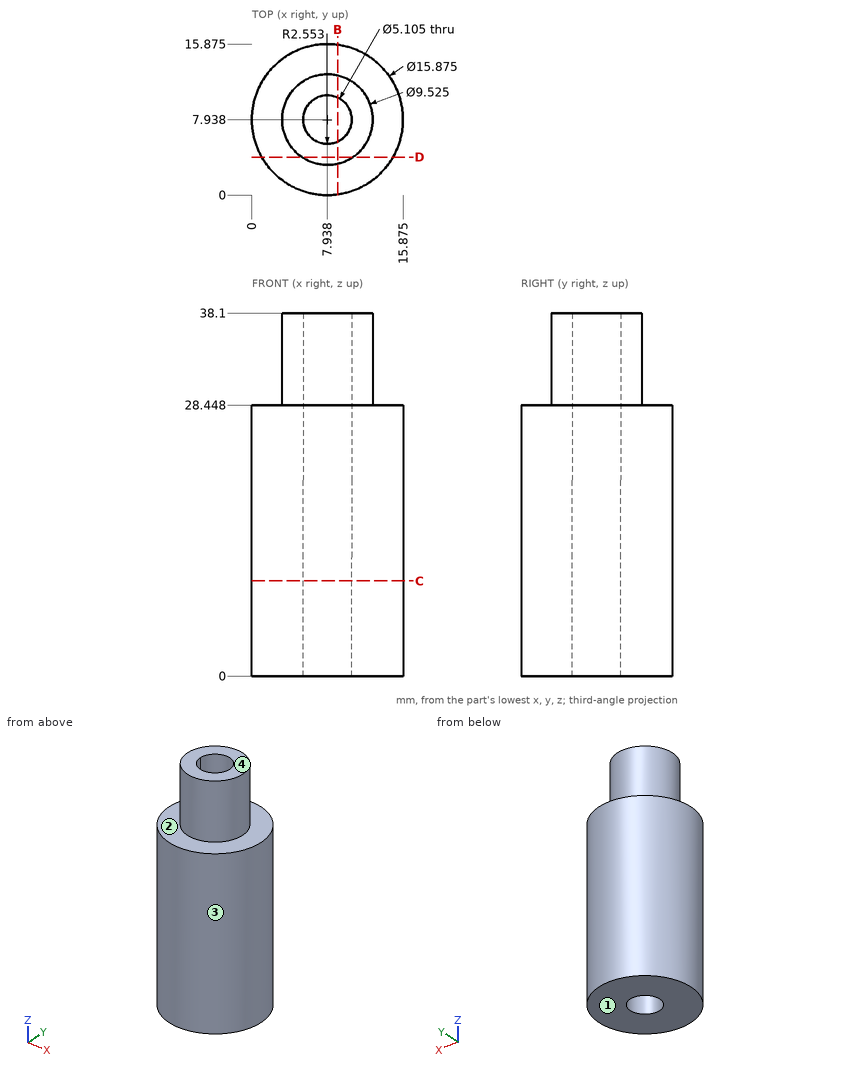
Part print with two shaded views. Sizes in mm from the minimum x, y, z corner. A direction names the side the tool comes from. Coordinates: 2 decimals unless noted, no trailing zeros. Write each loop counter-clockwise with the first axis right and the second up, starting at its lowest first coordinate (ties: lowest second). Pieces come first, ordered by that corner, then holes. Notation, with made-up numbers: (26, 5.25) - (72, 5.25) arc R14 ccw to (72, 25.25) - close; hole circle Ø11 at (78.25, 5.25). An arc over 180 degrees is marked (long way). Put each result on its own line as item: value.
1. Flat gauge pins, fed straight in: pin 1 Ø3 at (x, z) = (12, 28.5) entering from -Y (1 decimal); pin 2 Ø4 at (x, y) = (7.94, 7.94) entering from +Z; pin 3 Ø1.5 at (x, z) = (6, 24.5) entering from +Y (1 decimal). Where does each tip first touch, or does it go through?
Final values:
pin 1: stops at y = 0.4
pin 2: passes through
pin 3: stops at y = 15.8
2. Band-saw the part on D-D (y = 4). Write the cut outline in (x, z) (1 decimal).
Final values:
outline: (1, 0) - (14.8, 0) - (14.8, 28.4) - (10.6, 28.4) - (10.6, 38.1) - (5.3, 38.1) - (5.3, 28.4) - (1, 28.4) - close
3. Two-plate mould, pull along X, no slides. Class the marked faces 3 and 4: +X half, -X half, draft (parallel to the pull), parting line (faces both ways), or undercut.
Final values:
face 3: parting line
face 4: draft
4. Band-saw the part on C-C (z = 10). Write the cut outline in (x, y) (1 decimal).
Final values:
outline: circle Ø15.9 at (7.9, 7.9); hole circle Ø5.1 at (7.9, 7.9)
5. Band-saw the part on B-B (x = 9). Write the cut outline in (y, z) (1 decimal).
Final values:
outline: (0.1, 0) - (5.6, 0) - (5.6, 38.1) - (3.3, 38.1) - (3.3, 28.4) - (0.1, 28.4) - close; (10.3, 0) - (15.8, 0) - (15.8, 28.4) - (12.6, 28.4) - (12.6, 38.1) - (10.3, 38.1) - close
6. 3-axis set-ups, long thin cutter, end or side, ignore diameter. For the marked faces 1 and 2: which of +Z, -Z, +X, -X, +Y, -Y reach the whole face in a straight line?
Final values:
face 1: -Z, +X, -X, +Y, -Y
face 2: +Z
7. Probe line 1 along X through (y, z) = (7.75, 18.5); line 2 along Z through (x, y) = (2, 11.75); line 3 along Y through (x, z) = (8.25, 17) (1 decimal). List the from-to ranges inside material, lowest first. Write a range as [from, to].
Final values:
line 1: x = [0, 5.39], [10.48, 15.87]
line 2: z = [0, 28.45]
line 3: y = [0, 5.4], [10.5, 15.9]
